Work out the finished part from the listing and answer in its coordinate system (mm). Face numbers are marked on the shaded views. A direction names the side the tool comes from. Give positions to 0.01 mm unless a question says otherwise; leave off trailing zeros. Loops run counter-clockwise (first coordinate to the right, second up) from the corner with the lowest first, then second, coordinate; pieces in that order, holes last.
from build123d import *

# Parameters (mm, degrees)
SKETCH1_W                        = 127
SKETCH1_H                        = 152.4
BOSS_EXTRUDE1_DEPTH              = 12.7
SKETCH2_R                        = 14.2875
CUT_EXTRUDE1_DEPTH               = 13.7
FILLET1_R                        = 12.7
SKETCH3_W                        = 127
SKETCH3_H                        = 3.261499881
BOSS_EXTRUDE2_DEPTH              = 12.7
F_1_4_20_TAPPED_HOLE1_AT_2_COUNT = 2
F_1_4_20_TAPPED_HOLE1_AT_2_PITCH = 38.1
SKETCH6_W                        = 12.7
SKETCH6_H                        = 19.05
BOSS_EXTRUDE3_DEPTH              = 12.7
SKETCH7_R                        = 0.79375
CUT_EXTRUDE2_DEPTH               = 13.7


with BuildPart() as part:
    # Sketch1 → Boss-Extrude1 (new body)
    with BuildSketch(Plane.XY):
        with Locations((0, 76.2)):
            Rectangle(SKETCH1_W, SKETCH1_H)
    extrude(amount=BOSS_EXTRUDE1_DEPTH)

    # Sketch2 → Cut-Extrude1 (cut, through all)
    with BuildSketch(Plane.XY.offset(12.7)):
        with Locations((0, 95.25)):
            Circle(SKETCH2_R)
        with BuildLine():
            Line((31.75, 95.25), (31.75, 50.8))
            Line((31.75, 50.8), (63.5, 50.8))
            Line((63.5, 50.8), (63.5, 152.4))
            Line((63.5, 152.4), (-63.5, 152.4))
            Line((-63.5, 152.4), (-63.5, 50.8))
            Line((-63.5, 50.8), (-31.75, 50.8))
            Line((-31.75, 50.8), (-31.75, 95.25))
            ThreePointArc((-31.75, 95.25), (0, 127), (31.75, 95.25))
        make_face()
    extrude(amount=-CUT_EXTRUDE1_DEPTH, mode=Mode.SUBTRACT)

    # Fillet1
    fillet1_edges = [part.edges().sort_by_distance(p)[0] for p in [
        (-31.75, 50.8, 6.35),
        (31.75, 50.8, 6.35),
    ]]
    fillet(fillet1_edges, radius=FILLET1_R)

    # Sketch3 → Boss-Extrude2 (add)
    with BuildSketch(Plane.XY.offset(12.7)):
        with Locations((0, -1.630749941)):
            Rectangle(SKETCH3_W, SKETCH3_H)
    extrude(amount=-BOSS_EXTRUDE2_DEPTH)

    # Sketch4 → 1/4-20 Tapped Hole1 (revolve, cut)
    with BuildSketch(Plane(origin=(63.5, 42.81925006, 6.35), x_dir=(0, 0, -1), z_dir=(0, 1, 0))):
        Polygon((0, 0), (0, 18.043816902), (2.5527, 16.51), (2.5527, 0), align=None)
    f_1_4_20_tapped_hole1 = revolve(axis=Axis((69.85, 42.81925006, 6.35), (-1, 0, 0)), mode=Mode.SUBTRACT)

    # 1/4-20 Tapped Hole1 at 2: 1/4-20 Tapped Hole1 ×2
    with Locations(*[(0, -i * F_1_4_20_TAPPED_HOLE1_AT_2_PITCH, 0) for i in range(1, F_1_4_20_TAPPED_HOLE1_AT_2_COUNT)]):
        add(f_1_4_20_tapped_hole1, mode=Mode.SUBTRACT)

    # Sketch6 → Boss-Extrude3 (add)
    with BuildSketch(Plane(origin=(63.5, 0, 0), x_dir=(0, 0, -1), z_dir=(1, 0, 0))):
        with Locations((-6.35, 23.76925006)):
            Rectangle(SKETCH6_W, SKETCH6_H)
    boss_extrude3 = extrude(amount=BOSS_EXTRUDE3_DEPTH)

    # Sketch7 → Cut-Extrude2 (cut, through all)
    with BuildSketch(Plane.XY.offset(12.7)):
        with Locations((63.5, 34.08800006)):
            Circle(SKETCH7_R)
        with Locations((63.5, 13.45050006)):
            Circle(SKETCH7_R)
    cut_extrude2 = extrude(amount=-CUT_EXTRUDE2_DEPTH, mode=Mode.SUBTRACT)

    # Mirror1: Cut-Extrude2, Boss-Extrude3, 1/4-20 Tapped Hole1 across plane
    add(cut_extrude2.mirror(Plane(origin=(0, 0, 0), x_dir=(0, 0, 1), z_dir=(1, 0, 0))), mode=Mode.SUBTRACT)
    add(boss_extrude3.mirror(Plane(origin=(0, 0, 0), x_dir=(0, 0, 1), z_dir=(1, 0, 0))))
    add(f_1_4_20_tapped_hole1.mirror(Plane(origin=(0, 0, 0), x_dir=(0, 0, 1), z_dir=(1, 0, 0))), mode=Mode.SUBTRACT)

    # Mirror1 copy 1 sketch → Mirror1 copy 1 (revolve, cut)
    with BuildSketch(Plane(origin=(-63.5, 4.71925006, 6.35), x_dir=(0, 0, -1), z_dir=(0, 1, 0))):
        Polygon((0, 0), (0, -18.043816902), (2.5527, -16.51), (2.5527, 0), align=None)
    revolve(axis=Axis((-69.85, 4.71925006, 6.35), (-1, 0, 0)), mode=Mode.SUBTRACT)


solid = part.part
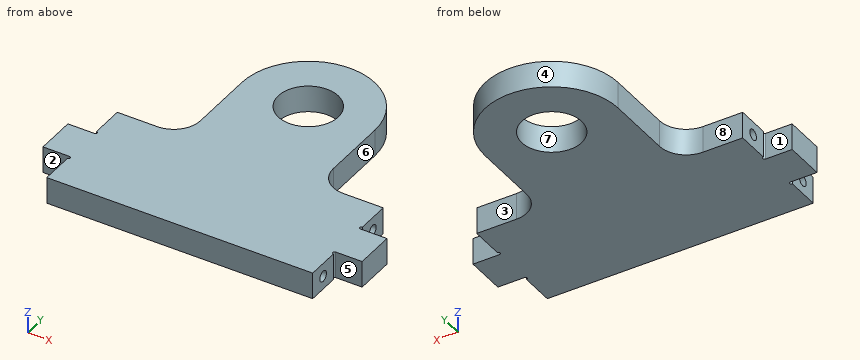
Item 1: For the marked faces 1, 2, 3, 4 and 5, determine the directions among +Z, -Z, +X, -X, +Y, -Y from which every point of the face is accessible in a straight line to the end or side of a thin tool.
Item 2: Consider line 1 (Y direction, x = -58.25, z = 6.35); line 2 (Y direction, x = 0, z = 9); line 3 (Y direction, x = 56, z = 4). Determine where each line is inside the solid, lowest interval first.
Item 3: Find section B-B, the plane y = 90.5. Write down the section's boundary in (x, z).
Item 4: Find section D-D, the plane y = 74. Write down the section's boundary in (x, z), plus the area to 3 significant figures.
Item 5: Determine the mould class of the marked faces 6, 7 and 8 for opening direction Y: released by +Y, released by -Y, zero draft, split by the parting line, or undercut.
Item 6: Find section C-C, the plane x = -51. Write down the section's boundary in (y, z), plus the area to 3 significant figures.
Item 7: Flat-ended cylindrical pins translate along their axes: pin 1 Ø4 at (y, z) = (8, 5.5) entering from +X; pin 2 Ø1.5 at (y, z) = (110.5, 9.5) entering from -X; pin 3 Ø6.5 at (y, z) = (40, 7.5) entering from -X. Find the tip coordinate at first contact, or state that the pin passes through.
Item 8: Find section A-A, the plane x = 0. Write down the section's boundary in (y, z), plus the area to 3 significant figures.
Ans:
1. face 1: +Z, -Z, -X, +Y
1. face 2: +Z, -Z, -X, -Y
1. face 3: +Z, -Z, +X, +Y
1. face 4: +Z, -Z, +Y
1. face 5: +Z, -Z, +X, -Y
2. line 1: y = -3.26 to 2.17, 7.27 to 40.27, 45.37 to 50.8
2. line 2: y = -3.26 to 80.96, 109.54 to 127
2. line 3: y = -3.26 to 3.72, 5.72 to 41.82, 43.82 to 50.8
3. outline: (-31.75, 0) - (-13.47, 0) - (-13.47, 12.7) - (-31.75, 12.7) - close; (13.47, 0) - (31.75, 0) - (31.75, 12.7) - (13.47, 12.7) - close
4. outline: (-31.75, 0) - (31.75, 0) - (31.75, 12.7) - (-31.75, 12.7) - close
4. area: 806 mm2
5. face 6: zero draft
5. face 7: undercut
5. face 8: released by +Y
6. outline: (-3.26, 0) - (50.8, 0) - (50.8, 12.7) - (-3.26, 12.7) - close; hole circle Ø5.11 at (4.72, 6.35); hole circle Ø5.11 at (42.82, 6.35)
6. area: 646 mm2
7. pin 1: stops at x = 63.5
7. pin 2: stops at x = -28.25
7. pin 3: stops at x = -63.5
8. outline: (-3.26, 0) - (80.96, 0) - (80.96, 12.7) - (-3.26, 12.7) - close; (109.54, 0) - (127, 0) - (127, 12.7) - (109.54, 12.7) - close
8. area: 1,290 mm2
